Verification items for the finished model (mm, model axes). Give positions to 0.01 mm unless a question says otherwise; leave off trailing zeros. Loops run counter-clockwise (first coordinate to the right, second up) from the corner with the lowest first, then second, coordinate; pieces in that order, holes last. Notation, with made-up numbers: (86, -16.5) -> (107, -16.5) arc R17 cw to (107, 13.5) -> close; hole circle Ø6 at (35.25, 16.5). An arc over 180 degrees is marked (long way). Answer in a Markdown table with one row per item. Add a question column.
Q1. Gauge pin test, flat ends, axial feed: P1, Ø4.5, axis at y = 0, z = 0, coming from the +X side; P2, Ø4, axis at x = 6.5, z = 2.5, coming from the +Y side; P3, Ø1.5, axis at x = 7, y = 1.5, coming from the +Z side. Record the tip position at first contact, or that the pin passes through.
Q2. Release check for a two-part mould opening along Y. For faces 1 (the face through (4.44, -1.08, -4.88)), 2 (the face through (5.69, -0.358, -2.727)), 3 (the face through (0, 4, -2)) record: pulls with the +Y half, pulls with the -Y half, needs draft (parallel to the pull), parting line crosses it, or undercut.
Q3. Section check A-A on x = 8. Enter the section's corners in (y, z), and give its area (3 significant figures).
Q4. Material ranges on probe 1 along Z at (x, y) = (7.5, 0); probe 2 along X at (y, z) = (1.25, -4); probe 3 along Y at (x, z) = (7.75, -0.75), recorded low to high.
Q5. Section check B-B on x = 9.5. Enter the section's corners in (y, z).
Autodesk Inventor part; units mm, degrees
ref_plane "YZ Plane" through (0, 0, 0) normal (1, 0, 0) x (0, 1, 0)
ref_plane "XZ Plane" through (0, 0, 0) normal (0, 1, 0) x (-1, 0, 0)
ref_plane "XY Plane" through (0, 0, 0) normal (0, 0, 1) x (1, 0, 0)
sketch "Skizze1" plane through (0, 0, 0) normal (0, 0, 1) x (1, 0, 0)
  line L0 (0, 2.75) -> (0, 5)
  line L1 (0, 5) -> (10, 5)
  line L2 (10, 5) -> (10, 2.75)
  line L3 (10, 2.75) -> (0, 2.75)
  line L4 (-9.5331, 0) -> (16.2451, 0)
  line L5 (-14.6887, 0) -> (21.4008, 0)
  line L6 (0, -0.7) -> (0, 4.2)
  dimension "d0" = 10
  dimension "d1" = 5.5
  dimension "d2" = 10
revolve "Körper" add sketch "Skizze1" angle 360 about axis through (-9.5331, 0, 0) along (1, 0, 0)
chamfer "Fase1" distance 1.25 angle 15 1 edges at (10, -5, 0) measured on face at (3.3333, 4.9353, -0.8021)
fillet "Rundung1" radius 1.5 1 edges at (0, -2.75, 0)
equation "\"d6\" = PHH"
equation "\"d7\" = ANG"
equation "\"d13\" = PHH"
equation "\"d11\" = RR"
equation "\"d0\" = SD2"
equation "\"d1\" = NND"
equation "\"d2\" = NLG"
equation "\"NLG\" = 10"
equation "\"NND\" = 5.5"
equation "\"SD2\" = 10"
equation "\"PHH\" = 1.25"
equation "\"ANG\" = 15deg"
equation "\"RR\" = 1.5"
equation "\"NNDMAX\" = 6"
equation "\"NNDMIN\" = 5.1"
equation "\"SEWI\" = 30deg"
properties part number "DIN 179 - A 5,5 x 10" material "Stahl, weich"
Taken from the geometry:
| question | item | result |
|---|---|---|
| 1 | P1 | passes through |
| 1 | P2 | stops at y = 4.97 |
| 1 | P3 | stops at z = 4.94 |
| 2 | face 1 | parting line crosses it |
| 2 | face 2 | undercut |
| 2 | face 3 | needs draft |
| 3 | outline | circle Ø10 at (0, 0); hole circle Ø5.5 at (0, 0) |
| 3 | area | 54.8 mm² |
| 4 | probe 1 | z = -5 to -2.75, 2.75 to 5 |
| 4 | probe 2 | x = 0 to 10 |
| 4 | probe 3 | y = -4.94 to -2.65, 2.65 to 4.94 |
| 5 | outline | circle Ø9.6 at (0, 0); hole circle Ø5.5 at (0, 0) |
